Build history of the part. All positions in model axes, mm. A direction names the side the tool comes from. Round coordinates to 2 decimals unless told otherwise and drop trailing zeros.
Item 1: Wall check: probe 1 along Y at (x, z) = (0, 0); probe 2 along X at (y, z) = (0, 19.25); probe 3 along Z at (x, y) = (2.5, -2.75). Give the ranges that are in metal, low to high.
Item 2: Mould opens along Z. For faces 6 (the cylindrical face through (-16.243, -1.802, 5.723)), 7 (the cylindrical face through (16.634, -2.703, 21.42)), 8 (the flat face through (-16.75, -6, -2)) say: +Z half, -Z half, draft (parallel to the pull), parting line (faces both ways), or undercut.
Item 3: Band-saw the part on B-B, the plane y = 2.75. Count the separate pieces of the cut face and the enclosed holes in it, then the cut area to 3 significant figures.
Item 4: 3-axis set-ups, long thin cutter, end or side, ignore diameter. For faces 1 (the cylindrical face through (-14.37, 5.78, -7.54)), 2 (the flat face through (33.85, 4, 2)), 3 (the flat face through (11, -5.4, 24.8)), 4 (the flat face through (6, -4, 25.8)), 5 (the cylindrical face through (25.04, -2.17, 9.76)): which of +Z, -Z, +X, -X, +Y, -Y reach the whole face in a straight line?
Item 5: Drop flat-ended pins along their axis: pin 1 Ø10 at (x, y) = (12.5, -2) entering from -Z; pin 2 Ø5 at (y, z) = (2, -2) entering from +X; pin 3 Ø6 at (x, z) = (28, 10.5) entering from -Y; pin 4 Ø1 at (x, z) = (14.5, -3) entering from -Y. Give the stop position or say it passes through.
```python
from build123d import *
from build123d.topology import SkipClean

# Parameters (mm, degrees)
SKETCH_2_R          = 8
SKETCH_2_R_2        = 4
EXTRUDE_1_DEPTH     = 26.1
SKETCH_4_R          = 8
EXTRUDE_2_DEPTH     = 13.05
SKETCH_6_R          = 4
CUT_EXTRUDE_1_DEPTH = 63.05
SKETCH_7_R          = 4
CUT_EXTRUDE_2_DEPTH = 25


with BuildPart() as part:
    # Эскиз1 → Повернуть1 (revolve)
    with BuildSketch(Plane.XY, mode=Mode.PRIVATE) as revolve_1_sk:
        Polygon((-16.75, -8), (-16.75, -6), (-15.75, -6), (-15.75, -8.75), (-15, -9.5), (-13.75, -9.5), (-13.75, -9), (-13, -9), (-13, -10), (-5, -10), (-5, -4), (-17.75, -4), (-17.75, -8), align=None)
    revolve(revolve_1_sk.sketch.rotate(Axis((-21.049489232, 0, 0), (1, 0, 0)), 270), axis=Axis((-21.049489232, 0, 0), (1, 0, 0)))

    # Эскиз2 → Бобышка-Вытянуть1 (add)
    with BuildSketch(Plane(origin=(-5, 0, 0), x_dir=(0, 0, -1), z_dir=(1, 0, 0))):
        with Locations(Location((0, 0, 0), (0, 0, 180))):
            Circle(SKETCH_2_R)
        with Locations(Location((0, 0, 0), (0, 0, 180))):
            Circle(SKETCH_2_R_2, mode=Mode.SUBTRACT)
    extrude(amount=EXTRUDE_1_DEPTH)

    # Эскиз3 → Повернуть2 (revolve)
    with SkipClean():  # the faces are left unmerged after this step: merging them gives an invalid solid
        with BuildSketch(Plane.XY):
            Polygon((32.85, 8), (32.85, 6), (31.85, 6), (31.85, 8.75), (31.1, 9.5), (29.85, 9.5), (29.85, 9), (29.1, 9), (29.1, 10), (21.1, 10), (21.1, 4), (33.85, 4), (33.85, 8), align=None)
        revolve(axis=Axis((47.149489232, 0, 0), (-1, 0, 0)))

    # Эскиз4 → Бобышка-Вытянуть2 (add)
    with SkipClean():  # the faces are left unmerged after this step: merging them gives an invalid solid
        with BuildSketch(Plane.XY):
            with Locations(Location((8.05, 0, 0), (0, 0, 90))):
                Circle(SKETCH_4_R)
        extrude(amount=EXTRUDE_2_DEPTH)

    # Эскиз5 → Повернуть3 (revolve)
    with SkipClean():  # the faces are left unmerged after this step: merging them gives an invalid solid
        with BuildSketch(Plane(origin=(0, 0, 0), x_dir=(1, 0, 0), z_dir=(0, 1, 0))):
            Polygon((16.05, -24.8), (14.05, -24.8), (14.05, -23.8), (16.8, -23.8), (17.55, -23.05), (17.55, -21.8), (17.05, -21.8), (17.05, -21.05), (18.05, -21.05), (18.05, -13.05), (12.05, -13.05), (12.05, -25.8), (16.05, -25.8), align=None)
        revolve(axis=Axis((8.05, 0, 29.099489232), (0, 0, -1)))

    # Эскиз6 → Вырез-Вытянуть1 (cut)
    with SkipClean():  # the faces are left unmerged after this step: merging them gives an invalid solid
        with BuildSketch(Plane.ZY.offset(17.75)):
            Circle(SKETCH_6_R)
        extrude(amount=-CUT_EXTRUDE_1_DEPTH, mode=Mode.SUBTRACT)

    # Эскиз7 → Вырез-Вытянуть2 (cut)
    with SkipClean():  # the faces are left unmerged after this step: merging them gives an invalid solid
        with BuildSketch(Plane.XY.offset(25.8)):
            with Locations((8.05, 0)):
                Circle(SKETCH_7_R)
        extrude(amount=-CUT_EXTRUDE_2_DEPTH, mode=Mode.SUBTRACT)


solid = part.part
```
Results:
1. probe 1: y = -8 to -4, 4 to 8
1. probe 2: x = -1.95 to 4.05, 12.05 to 18.05
1. probe 3: z = -7.51 to -2.9, 2.9 to 23.8, 24.8 to 25.8
2. face 6: parting line
2. face 7: undercut
2. face 8: draft
3. separate pieces: 3
3. enclosed holes: 0
3. area: 727 mm2
4. face 1: -X
4. face 2: +Z, -Z, +X, +Y, -Y
4. face 3: none
4. face 4: +Z, +X, -X, +Y, -Y
4. face 5: +X
5. pin 1: stops at z = -8
5. pin 2: stops at x = 33.85
5. pin 3: stops at y = -6.61
5. pin 4: stops at y = -7.6
